CAD build for the part. Positions are in the model's coordinates, mm. Face numbers are marked on the shaded views. A direction names the side the tool comes from. Give positions to 0.01 mm unless a question says otherwise; leave off trailing zeros. Loops run counter-clockwise (first coordinate to the right, second up) from the corner with the lowest first, then second, coordinate; pieces in that order, holes last. Notation, with made-up numbers: M 58.25,48 L 102.25,48 A10 ccw 102.25,61 Z; hole C 41,73.5 d3. An arc over 180 degrees is marked long. One line per question, with ' | ' between items.
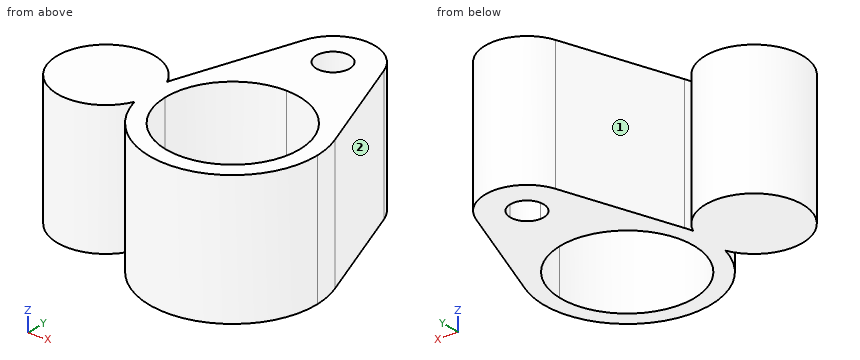
```python
from build123d import *

# Parameters (mm, degrees)
F2_DEPTH = 34.036


# Not quite as in the source:
# - a variable given as a bare number and used for a length is read in inches; the dataset says mm whatever the document's units were


with BuildPart() as f2:
    # F1 (on Top) → F2 (new body)
    with BuildSketch(Plane.XY):
        with BuildLine():
            ThreePointArc((-20.9431391397, -5.2452857858), (2.6425107354, -21.4276745592), (21.59, 0))
            ThreePointArc((21.59, 0), (21.2790729029, 3.6509117207), (20.3552472078, 7.1966666667))
            ThreePointArc((20.3552472078, 7.1966666667), (12.4649923156, 17.6281611796), (9.2e-09, 21.59))
            Line((0, 21.59), (0, 17.272))
            ThreePointArc((0, 17.272), (12.2131483247, 12.2131483247), (17.272, 0))
            ThreePointArc((17.272, 0), (0, -17.272), (-17.272, 0))
            Line((-17.272, 0), (-19.7981337132, 0))
            ThreePointArc((-19.7981337132, 0), (-20.0877162422, -2.6844021868), (-20.9431391397, -5.2452857858))
        make_face()
        with BuildLine():
            ThreePointArc((9.2e-09, 21.59), (12.4649923156, 17.6281611796), (20.3552472078, 7.1966666667))
            Line((20.3552472078, 7.1966666667), (10.1776236039, 35.9833333333))
            ThreePointArc((10.1776236039, 35.9833333333), (10.6395364515, 34.2104558603), (10.795, 32.385))
            ThreePointArc((10.795, 32.385), (7.6332177062, 24.7517823004), (9.2e-09, 21.59))
        make_face()
        with BuildLine():
            ThreePointArc((-20.9431391397, 5.2452857858), (-44.9718662868, 0), (-20.9431391397, -5.2452857858))
            ThreePointArc((-20.9431391397, -5.2452857858), (-21.4276745592, -2.6425107354), (-21.59, 0))
            ThreePointArc((-21.59, 0), (-21.4276745592, 2.6425107354), (-20.9431391397, 5.2452857858))
        make_face()
        with BuildLine():
            ThreePointArc((-21.59, 0), (-21.4276745592, -2.6425107354), (-20.9431391397, -5.2452857858))
            ThreePointArc((-20.9431391397, -5.2452857858), (-20.0877162422, -2.6844021868), (-19.7981337132, 0))
            Line((-19.7981337132, 0), (-21.59, 0))
        make_face()
        with BuildLine():
            Line((0, 17.272), (0, 21.59))
            ThreePointArc((9.2e-09, 21.59), (-12.464992308, 17.6281611849), (-20.3552472078, 7.1966666667))
            ThreePointArc((-20.3552472078, 7.1966666667), (-20.6722313881, 6.2279169422), (-20.9431391397, 5.2452857858))
            ThreePointArc((-20.9431391397, 5.2452857858), (-20.0877162422, 2.6844021868), (-19.7981337132, 0))
            Line((-19.7981337132, 0), (-17.272, 0))
            ThreePointArc((-17.272, 0), (-12.2131483247, 12.2131483247), (0, 17.272))
        make_face()
        with BuildLine():
            ThreePointArc((-20.3552472078, 7.1966666667), (-12.464992308, 17.6281611849), (9.2e-09, 21.59))
            ThreePointArc((9.2e-09, 21.59), (-8.8140805884, 26.1525038403), (-10.1776236039, 35.9833333333))
            Line((-10.1776236039, 35.9833333333), (-20.3552472078, 7.1966666667))
        make_face()
        with BuildLine():
            ThreePointArc((-10.1776236039, 35.9833333333), (-8.8140805884, 26.1525038403), (9.2e-09, 21.59))
            ThreePointArc((9.2e-09, 21.59), (7.6332177062, 24.7517823004), (10.795, 32.385))
            ThreePointArc((10.795, 32.385), (10.6395364515, 34.2104558603), (10.1776236039, 35.9833333333))
            ThreePointArc((10.1776236039, 35.9833333333), (0, 43.18), (-10.1776236039, 35.9833333333))
        make_face()
        with BuildLine():
            ThreePointArc((4.318, 32.385), (3.0532870812, 29.3317129188), (0, 28.067))
            ThreePointArc((0, 28.067), (-3.0532870812, 35.4382870812), (4.318, 32.385))
        make_face(mode=Mode.SUBTRACT)
        with BuildLine():
            ThreePointArc((-20.9431391397, 5.2452857858), (-21.4276745592, 2.6425107354), (-21.59, 0))
            Line((-21.59, 0), (-19.7981337132, 0))
            ThreePointArc((-19.7981337132, 0), (-20.0877162422, 2.6844021868), (-20.9431391397, 5.2452857858))
        make_face()
    extrude(amount=F2_DEPTH)


solid = f2.part
```
Item 1: Saw through at D-D on z = 16. Give the cut face in (x, y) (3 decimals), and give its area (3 significant figures).
Conclusion:
outline: M -20.943,-5.245 A21.59 ccw long 20.355,7.197 L 10.178,35.983 A10.795 ccw -10.178,35.983 L -20.355,7.197 A21.59 ccw -20.943,5.245 A12.587 ccw long Z; hole C 0,0 d34.544; hole C 0,32.385 d8.636 | area: 1,510 mm²
Item 2: Drill centre lines: line 1 along Y through (x, z) = (0, 23); line 2 along X through (y, z) = (-8, 18.5); line 3 along X through (y, z) = (-10.5, 17). Where is each one in solid material? Low to high. Write a range as [from, to].
Conclusion:
line 1: [-21.59, -17.27], [17.27, 28.07], [36.7, 43.18] | line 2: [-42.1, -22.67], [-20.05, -15.31], [15.31, 20.05] | line 3: [-39.33, -25.44], [-18.86, -13.71], [13.71, 18.86]
Item 3: Drop flat-ended pins along their axis: P1, Ø4, axis at y = 15, z = 22.5, coming from the -X side; P2, Ø10, axis at y = 19, z = 13.5, coming from the -X side; P3, Ø3, axis at x = -23, z = 14, coming from the -Y side. Give the stop position or say it passes through.
Conclusion:
P1: x = -18.3 | P2: x = -17.95 | P3: y = -9.81
Item 4: Saw through at A-A on x = 13.5. Give the cut face in (y, z).
Conclusion:
outline: M -16.85,0 L -10.77,0 L -10.77,34.04 L -16.85,34.04 Z; M 10.77,0 L 26.59,0 L 26.59,34.04 L 10.77,34.04 Z
Item 5: 3-axis set-ups, long thin cutter, end or side, ignore diameter. For the marked faces 1 and 2: which of +Z, -Z, +X, -X, +Y, -Y reach the whole face in a straight line?
Conclusion:
face 1: +Z, -Z, +Y | face 2: +Z, -Z, +X, +Y
Item 6: Saw through at C-C on x = -1. Give the cut face in (y, z).
Conclusion:
outline: M -21.57,0 L -17.24,0 L -17.24,34.04 L -21.57,34.04 Z; M 17.24,0 L 28.18,0 L 28.18,34.04 L 17.24,34.04 Z; M 36.59,0 L 43.13,0 L 43.13,34.04 L 36.59,34.04 Z
Item 7: Saw through at B-B on y = 16. Give the cut face in (x, z).
Conclusion:
outline: M -17.24,0 L -6.51,0 L -6.51,34.04 L -17.24,34.04 Z; M 6.51,0 L 17.24,0 L 17.24,34.04 L 6.51,34.04 Z
